```python
from build123d import *

# Parameters (mm, degrees)
F0_W     = 31.75
F0_H     = 31.75
F0_W_2   = 25.654
F0_H_2   = 25.654
F1_DEPTH = 558.8
F3_D     = 9.525
F3_DEPTH = 12.7


with BuildPart() as f1:
    # F0 (on Front) → F1 (new body)
    with BuildSketch(Plane.XZ):
        with Locations((-41.375973, 31.78728)):
            Rectangle(F0_W, F0_H)
        with Locations((-41.375973, 31.78728)):
            Rectangle(F0_W_2, F0_H_2, mode=Mode.SUBTRACT)
    extrude(amount=F1_DEPTH)

    # F3
    with Locations(Plane.XY.offset(47.66228)):
        with Locations((-41.375973, -508), (-41.375973, -457.2), (-41.375973, -406.4), (-41.375973, -355.6), (-41.375973, -304.8), (-41.375973, -254)):
            Hole(F3_D / 2, depth=F3_DEPTH)


solid = f1.part
```
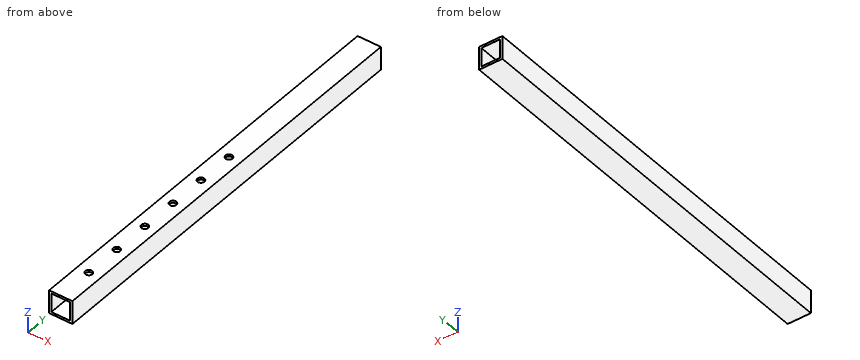
Could you check a few things on this model? Use its own coordinates, in mm. Round coordinates to 2 decimals unless told otherwise and drop trailing zeros. Write each loop counter-clockwise with the first axis right and the second up, starting at its lowest first coordinate (ties: lowest second). Pieces come first, ordered by that corner, then holes. Notation, with made-up numbers: M 37.25,14.25 L 79.25,14.25 A15 cw 79.25,23.25 Z; hole C -29.5,-32.5 d11. An arc over 180 degrees is marked long. Answer in a Markdown table with one row per item. Add a question column.
Q1. If I drill on line 1 (Z direction, x = -33, y = -371); line 2 (X direction, y = -317, z = 42.5); line 3 (X direction, y = -406, z = 46), over which ranges is the centre line in solid material (lowest first)? Write a range as from..to.
Q2. Imagine slicing it at B-B (y = -291.5). Please give me the cut outline in (x, z).
Q3. Imagine slicing it at A-A (z = 39). Please give me the cut outline in (x, y), then the cut area to 3 significant figures.
Q4. Imagine slicing it at C-C (y = -406.4). Please give me the cut outline in (x, z), then the cut area to 3 significant figures.
Values:
| question | item | result |
|---|---|---|
| 1 | line 1 | 15.91..18.96, 44.61..47.66 |
| 1 | line 2 | -57.25..-54.2, -28.55..-25.5 |
| 1 | line 3 | -57.25..-46.12, -36.63..-25.5 |
| 2 | outline | M -57.25,15.91 L -25.5,15.91 L -25.5,47.66 L -57.25,47.66 Z; hole M -54.2,18.96 L -28.55,18.96 L -28.55,44.61 L -54.2,44.61 Z |
| 3 | outline | M -57.25,-558.8 L -54.2,-558.8 L -54.2,0 L -57.25,0 Z; M -28.55,-558.8 L -25.5,-558.8 L -25.5,0 L -28.55,0 Z |
| 3 | area | 3,410 mm^2 |
| 4 | outline | M -57.25,15.91 L -25.5,15.91 L -25.5,47.66 L -36.61,47.66 L -36.61,44.61 L -28.55,44.61 L -28.55,18.96 L -54.2,18.96 L -54.2,44.61 L -46.14,44.61 L -46.14,47.66 L -57.25,47.66 Z |
| 4 | area | 321 mm^2 |
